Check sheet for the modelled part. Datum: model origin and axes. Units: mm. Coordinates: 2 decimals unless noted, no trailing zeros. Loops run counter-clockwise (first coordinate to the right, second up) from the corner with the lowest first, then second, coordinate; pieces in that order, holes last.
```python
from build123d import *

# Parameters (mm, degrees)
SKETCH1_R           = 1.7
BOSS_EXTRUDE1_DEPTH = 5
SKETCH2_W           = 4
SKETCH2_H           = 5
BOSS_EXTRUDE2_DEPTH = 42
SKETCH3_R           = 1.7
CUT_EXTRUDE1_DEPTH  = 69.75
FILLET1_R           = 10
FILLET2_R           = 10


with BuildPart() as part:
    # Sketch1 → Boss-Extrude1 (new body)
    with BuildSketch(Plane.XY):
        with BuildLine():
            Line((-49.959983987, 2), (49.959983987, 2))
            ThreePointArc((49.959983987, 2), (45.578077054, -20.558183092), (31.568754239, -38.773879814))
            Line((31.568754239, -38.773879814), (-31.568754239, -38.773879814))
            ThreePointArc((-31.568754239, -38.773879814), (-45.578077054, -20.558183092), (-49.959983987, 2))
        make_face()
        with Locations((-16, -3)):
            Circle(SKETCH1_R, mode=Mode.SUBTRACT)
        with Locations((16, -3)):
            Circle(SKETCH1_R, mode=Mode.SUBTRACT)
        with BuildLine():
            ThreePointArc((-44.4, -3), (-36.081832586, -23.081832586), (-16, -31.4))
            ThreePointArc((-16, -31.4), (-14.3, -29.7), (-16, -28))
            ThreePointArc((-16, -28), (-33.67766953, -20.67766953), (-41, -3))
            ThreePointArc((-41, -3), (-42.7, -1.3), (-44.4, -3))
        make_face(mode=Mode.SUBTRACT)
        with BuildLine():
            ThreePointArc((16, -31.4), (36.081832586, -23.081832586), (44.4, -3))
            ThreePointArc((44.4, -3), (42.7, -1.3), (41, -3))
            ThreePointArc((41, -3), (33.67766953, -20.67766953), (16, -28))
            ThreePointArc((16, -28), (14.3, -29.7), (16, -31.4))
        make_face(mode=Mode.SUBTRACT)
    extrude(amount=-BOSS_EXTRUDE1_DEPTH)

    # Sketch2 → Boss-Extrude2 (add)
    with BuildSketch(Plane(origin=(0, 2, 0), x_dir=(1, 0, 0), z_dir=(0, 1, 0))):
        with Locations((16.75, 2.5)):
            Rectangle(SKETCH2_W, SKETCH2_H)
        with Locations((-16.75, 2.5)):
            Rectangle(SKETCH2_W, SKETCH2_H)
    extrude(amount=BOSS_EXTRUDE2_DEPTH)

    # Sketch3 → Cut-Extrude1 (cut, through all)
    with BuildSketch(Plane(origin=(18.75, 0, 0), x_dir=(0, 0, -1), z_dir=(1, 0, 0))):
        with Locations((2.5, 40)):
            Circle(SKETCH3_R)
        with Locations((2.5, 18.3)):
            Circle(SKETCH3_R)
    extrude(amount=-CUT_EXTRUDE1_DEPTH, mode=Mode.SUBTRACT)

    # Fillet1
    fillet1_edges = [part.edges().sort_by_distance(p)[0] for p in [
        (31.568754239, -38.773879814, -2.5),
    ]]
    fillet(fillet1_edges, radius=FILLET1_R)

    # Fillet2
    fillet2_edges = [part.edges().sort_by_distance(p)[0] for p in [
        (-31.568754239, -38.773879814, -2.5),
    ]]
    fillet(fillet2_edges, radius=FILLET2_R)


solid = part.part
```
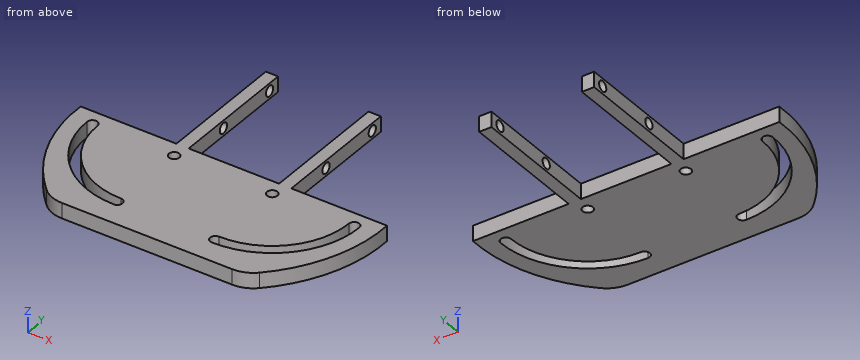
1) Section check A-A on y = 40. Enter the section's corners in (x, z).
Answer sheet:
outline: (-18.75, -5) - (-14.75, -5) - (-14.75, -4.2) - (-18.75, -4.2) - close; (-18.75, -0.8) - (-14.75, -0.8) - (-14.75, 0) - (-18.75, 0) - close; (14.75, -5) - (18.75, -5) - (18.75, -4.2) - (14.75, -4.2) - close; (14.75, -0.8) - (18.75, -0.8) - (18.75, 0) - (14.75, 0) - close
2) Scan lines: line 1 (Y direction, x = -15.95, z = -2.5); line 2 (X direction, y = 21, z = -2.85); line 3 (Y direction, x = -16, z = -0.45). Record each from-to range of solid material in increasing order.
Answer sheet:
line 1: y = -38.77 to -31.4, -28 to -4.7, -1.3 to 16.6, 20 to 38.3, 41.7 to 44
line 2: x = -18.75 to -14.75, 14.75 to 18.75
line 3: y = -38.77 to -31.4, -28 to -4.7, -1.3 to 44
3) Section check C-C on x = -42.7. Enter the section's corners in (y, z), plus the area to 3 significant figures.
Answer sheet:
outline: (-26.01, -5) - (-12.68, -5) - (-12.68, 0) - (-26.01, 0) - close; (-1.3, -5) - (2, -5) - (2, 0) - (-1.3, 0) - close
area: 83.2 mm2
4) Section check D-D on y = -10. Enter the section's corners in (x, z), plus the area to 3 significant figures.
Answer sheet:
outline: (-48.99, -5) - (-43.52, -5) - (-43.52, 0) - (-48.99, 0) - close; (-40, -5) - (40, -5) - (40, 0) - (-40, 0) - close; (43.52, -5) - (48.99, -5) - (48.99, 0) - (43.52, 0) - close
area: 455 mm2
5) Section check B-B on z = -3.3. Give the number of separate pieces and of enclosed holes in the cut face, plus the area to 3 significant figures.
Answer sheet:
separate pieces: 5
enclosed holes: 4
area: 3,610 mm2
6) Depth check by flat-ended pin: pin 1 (1 mm diameter, centred on y = 21.5, z = -3, fed in from -X); pin 2 (2.5 mm diameter, centred on x = 16, y = -3, fed in from -Z); pin 3 (1 mm diameter, centred on y = -15.5, z = -3, fed in from -X); pin 4 (3 mm diameter, centred on y = 2.5, z = -4, fed in from +X). Enter the tip coordinate at first touch or a pass-through.
Answer sheet:
pin 1: stops at x = -18.75
pin 2: passes through
pin 3: stops at x = -47.7
pin 4: stops at x = 49.99
